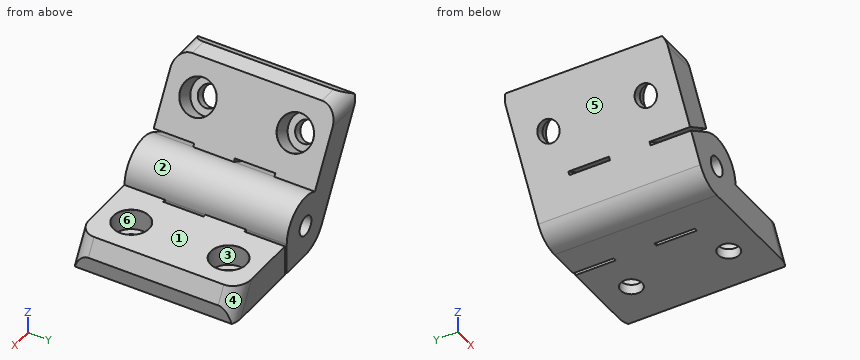
from build123d import *

# Parameters (mm, degrees)
SKETCH_9_R                  = 3
EXTRUDE_4_DEPTH             = 25
EXTRUDE_4_DEPTH_BACK        = 25
EXTRUDE_5_REACH             = 27
SKETCH_10_R                 = 3
EXTRUDE_5_DIRECTION_2_REACH = 27
HOLE_WIZARD_M61_AT_2_COUNT  = 2
HOLE_WIZARD_M61_AT_2_PITCH  = 30
HOLE_WIZARD_M62_AT_2_COUNT  = 2
HOLE_WIZARD_M62_AT_2_PITCH  = 30
CHAMFER_1_SIZE              = 5
CHAMFER_1_SIZE2             = 2.886751346
CHAMFER_1_PART_2_SIZE       = 5
CHAMFER_1_PART_2_SIZE2      = 2.886751346
SKETCH_15_W                 = 1
SKETCH_15_H                 = 12.5
CUT_EXTRUDE_1_DEPTH         = 10.5
SKETCH_16_W                 = 1
SKETCH_16_H                 = 12.5
CUT_EXTRUDE_2_DEPTH         = 28.463457268
FILLET_2_R                  = 5


with BuildPart() as part:
    # Sketch 9 → Extrude 4 (new body, two sides)
    with BuildSketch(Plane(origin=(0, 0, 0), x_dir=(1, 0, 0), z_dir=(0, 1, 0))) as extrude_4_sk:
        with BuildLine():
            Line((0, 9.5), (36, 9.5))
            Line((36, 9.5), (36, 0))
            Line((36, 0), (9.5, 0))
            ThreePointArc((9.5, 0), (-6.717514421, -6.717514421), (0, 9.5))
        make_face()
        with Locations(Location((0, 0, 0), (0, 0, 270))):  # turned: the seam where the file's is
            Circle(SKETCH_9_R, mode=Mode.SUBTRACT)
    extrude(amount=EXTRUDE_4_DEPTH)
    extrude(extrude_4_sk.sketch, amount=-EXTRUDE_4_DEPTH_BACK)

    # Extrude 5: up to this face of the body (flat: up to its plane)
    extrude_5_end = Plane(part.part.faces().sort_by_distance((11.152200141, 25, -2.543273154))[0])
    # Sketch 10 → Extrude 5 (add, up to the picked face)
    with BuildSketch(Plane(origin=(0, 0, 0), x_dir=(1, 0, 0), z_dir=(0, 1, 0)), mode=Mode.PRIVATE) as extrude_5_sk1:
        with BuildLine():
            Line((-8.227241336, 4.75), (-26.227241336, -26.426914536))
            Line((-26.227241336, -26.426914536), (-18, -31.176914536))
            Line((-18, -31.176914536), (-4.75, -8.227241336))
            ThreePointArc((-4.75, -8.227241336), (9.17629535, 2.458780928), (-8.227241336, 4.75))
        make_face()
        with Locations(Location((0, 0, 0), (0, 0, 270))):  # turned: the seam where the file's is
            Circle(SKETCH_10_R, mode=Mode.SUBTRACT)
    extrude_5_tool1 = split(extrude(extrude_5_sk1.sketch, amount=EXTRUDE_5_REACH, mode=Mode.PRIVATE), bisect_by=extrude_5_end, keep=Keep.BOTH, mode=Mode.PRIVATE)
    add(extrude_5_tool1.solids().sort_by(Axis((-7.778639, 0, 8.386452), (0, 1, 0)))[0])

    # Extrude 5 direction 2: up to this face of the body (flat: up to its plane)
    extrude_5_direction_2_end = Plane(part.part.faces().sort_by_distance((11.152200141, -25, -2.543273154))[0])
    # Sketch 10 → Extrude 5 direction 2 (add, up to the picked face)
    with BuildSketch(Plane(origin=(0, 0, 0), x_dir=(1, 0, 0), z_dir=(0, 1, 0)), mode=Mode.PRIVATE) as extrude_5_direction_2_sk1:
        with BuildLine():
            Line((-8.227241336, 4.75), (-26.227241336, -26.426914536))
            Line((-26.227241336, -26.426914536), (-18, -31.176914536))
            Line((-18, -31.176914536), (-4.75, -8.227241336))
            ThreePointArc((-4.75, -8.227241336), (9.17629535, 2.458780928), (-8.227241336, 4.75))
        make_face()
        with Locations(Location((0, 0, 0), (0, 0, 270))):  # turned: the seam where the file's is
            Circle(SKETCH_10_R, mode=Mode.SUBTRACT)
    extrude_5_direction_2_tool1 = split(extrude(extrude_5_direction_2_sk1.sketch, amount=-EXTRUDE_5_DIRECTION_2_REACH, mode=Mode.PRIVATE), bisect_by=extrude_5_direction_2_end, keep=Keep.BOTH, mode=Mode.PRIVATE)
    add(extrude_5_direction_2_tool1.solids().sort_by(Axis((-7.778639, 0, 8.386452), (0, -1, 0)))[0])

    # Sketch 12 → Hole Wizard M61 (revolve, cut)
    with BuildSketch(Plane(origin=(22.5, 15, 0), x_dir=(0, -1, 0), z_dir=(1, 0, 0))):
        Polygon((0, 0), (0, 9.5), (3.3, 9.5), (3.3, 6.4), (5.5, 6.4), (5.5, 0.025), (5.525, 0), align=None)
    hole_wizard_m61 = revolve(axis=Axis((22.5, 15, 6.35), (0, 0, -1)), mode=Mode.SUBTRACT)

    # Hole Wizard M61 at 2: Hole Wizard M61 ×2
    with Locations(*[(0, -i * HOLE_WIZARD_M61_AT_2_PITCH, 0) for i in range(1, HOLE_WIZARD_M61_AT_2_COUNT)]):
        add(hole_wizard_m61, mode=Mode.SUBTRACT)

    # Sketch 14 → Hole Wizard M62 (revolve, cut)
    with BuildSketch(Plane(origin=(-11.25, 15, 19.485571585), x_dir=(0.5, 0, -0.866025404), z_dir=(0, 1, 0))):
        Polygon((0, 0), (0, 27.463457268), (3.3, 27.463457268), (3.3, 6.4), (5.5, 6.4), (5.5, 0.025), (5.525, 0), align=None)
    hole_wizard_m62 = revolve(axis=Axis((-5.750738686, 15, 22.660571585), (-0.866025404, 0, -0.5)), mode=Mode.SUBTRACT)

    # Hole Wizard M62 at 2: Hole Wizard M62 ×2
    with Locations(*[(0, -i * HOLE_WIZARD_M62_AT_2_PITCH, 0) for i in range(1, HOLE_WIZARD_M62_AT_2_COUNT)]):
        add(hole_wizard_m62, mode=Mode.SUBTRACT)

    # Chamfer 1
    chamfer_1_edges = [part.edges().sort_by_distance(p)[0] for p in [
        (-18, 0, 31.176914536),
    ]]
    chamfer_1_side = [part.faces().sort_by_distance(p)[0] for p in [
        (-22.113620668, 0, 28.801914536),
    ]]
    chamfer(chamfer_1_edges, length=CHAMFER_1_SIZE, length2=CHAMFER_1_SIZE2, reference=chamfer_1_side[0])

    # Chamfer 1 part 2
    chamfer_1_part_2_edges = [part.edges().sort_by_distance(p)[0] for p in [
        (36, 0, 0),
    ]]
    chamfer_1_part_2_side = [part.faces().sort_by_distance(p)[0] for p in [
        (36, 0, -4.75),
    ]]
    chamfer(chamfer_1_part_2_edges, length=CHAMFER_1_PART_2_SIZE, length2=CHAMFER_1_PART_2_SIZE2, reference=chamfer_1_part_2_side[0])

    # Sketch 15 → Cut-Extrude 1 (cut, through all)
    with BuildSketch(Plane.XY):
        with Locations((10, 18.75)):
            Rectangle(SKETCH_15_W, SKETCH_15_H)
        with Locations((10, -6.25)):
            Rectangle(SKETCH_15_W, SKETCH_15_H)
    extrude(amount=-CUT_EXTRUDE_1_DEPTH, mode=Mode.SUBTRACT)

    # Sketch 16 → Cut-Extrude 2 (cut, through all)
    with BuildSketch(Plane(origin=(0, 0, 0), x_dir=(0.5, 0, -0.866025404), z_dir=(0.866025404, 0, 0.5))):
        with Locations((-10, -18.75)):
            Rectangle(SKETCH_16_W, SKETCH_16_H)
        with Locations((-10, 6.25)):
            Rectangle(SKETCH_16_W, SKETCH_16_H)
    extrude(amount=-CUT_EXTRUDE_2_DEPTH, mode=Mode.SUBTRACT)

    # Fillet 2
    fillet_2_edges = [part.edges().sort_by_distance(p)[0] for p in [
        (34.556624327, 25, -2.5),
        (34.556624327, -25, -2.5),
        (-19.443375673, 25, 28.676914536),
        (-19.443375673, -25, 28.676914536),
    ]]
    fillet(fillet_2_edges, radius=FILLET_2_R)


solid = part.part
Here's how the part is built. I have some questions about the finished solid (model axes, mm). Face numbers are marked on the shaded views. A direction names the side the tool comes from. Give positions to 0.01 mm unless a question says otherwise; leave off trailing zeros. Write each loop counter-clockwise with the first axis right and the second up, starting at its lowest first coordinate (ties: lowest second). Pieces come first, ordered by that corner, then holes. Notation, with made-up numbers: (20, 35) -> (44, 35) arc R16 ccw to (44, 41) -> close; hole circle Ø8 at (17.5, -13). An arc over 180 degrees is marked (long way). Use one line per item in the form item = value. Start each with the question number.
1. On a 3-axis mill with a long thin cutter (end or side, diameter ignored), from which of +Z, -Z, +X, -X, +Y, -Y can I reach the whole of each face in a straight line? I mean the marked faces 1 and 2. Say none if no direction works.
2. Imagine slicing it at A-A on x = 22.5. List the corners of the cut face in (y, z) for me (3 decimals).
3. If I drill on L1, parallel to Y at x = 22.5, z = -8.2; L2, parallel to Y at x = 23, z = -3.5; L3, parallel to X at y = 15, z = -3.5, over which ranges is the centre line in solid material (lowest first)?
4. Imagine slicing it at B-B on y = -15. State how many separate pieces and enclosed holes the cut face has, plus the area to 3 significant figures.
5. Will these pins go through, and if not, where does the flat tip stop? pin 1 Ø6 at (x, y) = (13, -17.5) entering from +Z; pin 2 Ø3 at (x, y) = (-5.5, 7.5) entering from +Z; pin 3 Ø5 at (y, z) = (-8.5, -2.5) entering from -X; pin 4 Ø6 at (x, y) = (22.5, 15) entering from -Z.
6. Imagine slicing it at D-D on x = 6.5. List the corners of the cut face in (y, z) for me, plus the area to 3 significant figures.
7. Imagine slicing it at C-C on y = 22.5. List the corners of the cut face in (x, z) for me.
8. Thinking about a two-plate mould opening in X: for the marked faces 3, 4, 5 and 6, which applies, +X half, -X half, draft (parallel to the pull), parting line (faces both ways), or undercut?
Entries:
q1.face_1 = +Z, +X, +Y, -Y
q1.face_2 = +Z, +Y, -Y
q2.outline = (-25, -9.5) -> (-18.3, -9.5) -> (-18.3, -6.4) -> (-20.5, -6.4) -> (-20.5, -0.025) -> (-20.525, 0) -> (-25, 0) -> close; (-11.7, -9.5) -> (11.7, -9.5) -> (11.7, -6.4) -> (9.5, -6.4) -> (9.5, -0.025) -> (9.475, 0) -> (-9.475, 0) -> (-9.5, -0.025) -> (-9.5, -6.4) -> (-11.7, -6.4) -> close; (18.3, -9.5) -> (25, -9.5) -> (25, 0) -> (20.525, 0) -> (20.5, -0.025) -> (20.5, -6.4) -> (18.3, -6.4) -> close
q3.L1 = -25 to -18.3, -11.7 to 11.7, 18.3 to 25
q3.L2 = -25 to -20.48, -9.52 to 9.52, 20.48 to 25
q3.L3 = -8.95 to 9.5, 10.5 to 17, 28 to 35.13
q4.separate_pieces = 4
q4.enclosed_holes = 1
q4.area = 592 mm²
q5.pin_1 = 0
q5.pin_2 = 12.12
q5.pin_3 = -10.97
q5.pin_4 = through
q6.outline = (-25, -9.5) -> (25, -9.5) -> (25, 6.93) -> (-25, 6.93) -> close
q6.area = 821 mm²
q7.outline = (-26.23, 26.43) -> (-8.23, -4.75) arc R9.5 ccw to (0, -9.5) -> (9.5, -9.5) -> (9.5, 0) arc R9.5 ccw to (-4.75, 8.23) -> (-16.17, 28.01) -> (-23.49, 28.01) -> close; (10.5, -9.5) -> (36, -9.5) -> (36, -6.34) -> (32.34, 0) -> (10.5, 0) -> close; hole circle Ø6 at (0, 0)
q8.face_3 = undercut
q8.face_4 = +X half
q8.face_5 = -X half
q8.face_6 = undercut
